from build123d import *

# Parameters (mm, degrees)
BOSS_EXTRUDE2_DEPTH = 6.096


with BuildPart() as part:
    # Sketch1 → Boss-Extrude2 (new body)
    with BuildSketch(Plane.XY):
        with BuildLine():
            Line((-4.0259, 0.692415095), (-4.0259, -1.7018))
            ThreePointArc((-4.0259, -1.7018), (-3.058766591, -4.036666591), (-0.7239, -5.0038))
            Line((-0.7239, -5.0038), (0.7239, -5.0038))
            ThreePointArc((0.7239, -5.0038), (3.058766591, -4.036666591), (4.0259, -1.7018))
            Line((4.0259, -1.7018), (4.0259, 0.692415095))
            ThreePointArc((4.0259, 0.692415095), (3.977581548, 1.682110135), (3.833085773, 2.662391684))
            add(Edge.make_bspline(
                [(3.833085773, 2.662391684), (2.882993145, 7.469428366), (1.294052888, 17.736271143), (0.32760263, 29.308652747), (0, 35.421228256)],
                knots=[0.032373922, 0.032373922, 0.032373922, 0.032373922, 0.516186961, 1, 1, 1, 1], degree=3))
            add(Edge.make_bspline(
                [(-3.833085773, 2.662391684), (-2.882993145, 7.469428366), (-1.294052888, 17.736271143), (-0.32760263, 29.308652747), (0, 35.421228256)],
                knots=[0.032373922, 0.032373922, 0.032373922, 0.032373922, 0.516186961, 1, 1, 1, 1], degree=3))
            ThreePointArc((-3.833085773, 2.662391684), (-3.977581548, 1.682110135), (-4.0259, 0.692415095))
        make_face()
        with BuildLine():
            Line((-1.7399, 1.7018), (-1.7399, -1.7018))
            ThreePointArc((-1.7399, -1.7018), (-1.44232049, -2.42022049), (-0.7239, -2.7178))
            Line((-0.7239, -2.7178), (0.7239, -2.7178))
            ThreePointArc((0.7239, -2.7178), (1.44232049, -2.42022049), (1.7399, -1.7018))
            Line((1.7399, -1.7018), (1.7399, 1.7018))
            ThreePointArc((1.7399, 1.7018), (1.44232049, 2.42022049), (0.7239, 2.7178))
            Line((0.7239, 2.7178), (-0.7239, 2.7178))
            ThreePointArc((-0.7239, 2.7178), (-1.44232049, 2.42022049), (-1.7399, 1.7018))
        make_face(mode=Mode.SUBTRACT)
    extrude(amount=BOSS_EXTRUDE2_DEPTH)


solid = part.part
The model under review builds one solid part; all positions refer to its coordinate system, in mm. A direction names the side the tool comes from. Coordinates: 2 decimals unless noted, no trailing zeros. Answer in a Markdown table with one row per item.
(1) Machinability: for faces 1 (the flat face through (0, 11, 6.096)), 2 (the flat face through (0, 2.718, 3)), which of the approach directions +Z, -Z, +X, -X, +Y, -Y give a long, thin tool a straight path to every point of the face, cutting with its end or side? Answer none if there is none.
Answers:
| item | result |
|---|---|
| face 1 | +Z, +X, -X, +Y, -Y |
| face 2 | +Z, -Z |
(2) Wall thickness on line 1 along X through (y, z) = (1, 5.75); line 2 along X through (y, z) = (16, 3.5); line 3 along X through (y, z) = (20.5, 0.5): over which ranges is each line inside the solid? List them lowest first.
Answers:
| item | result |
|---|---|
| line 1 | -4.02 to -1.74, 1.74 to 4.02 |
| line 2 | -1.7 to 1.7 |
| line 3 | -1.18 to 1.18 |
(3) Insertion check: pin 1 (1 mm diameter, centred on x = -2.5, z = 0.5, fed in from -Y); pin 2 (2 mm diameter, centred on y = 29.5, z = 4, fed in from +X); pin 3 (1 mm diameter, centred on y = 22, z = 5.5, fed in from -X). Each pin has a flat end and moves straight along its axis. Give the tip position at first contact, or say it passes through.
Answers:
| item | result |
|---|---|
| pin 1 | y = -4.75 |
| pin 2 | x = 0.45 |
| pin 3 | x = -1.07 |
(4) The part is to be moulded in two halves that separate along X. For faces 3 (the cylindrical face through (-3.976, 1.696, 3.005)), 4 (the flat face through (-1.74, 0, 3)), 5 (the flat face through (0, -5.004, 3)), say which applies: +X half, -X half, draft (parallel to the pull), parting line (faces both ways), or undercut.
Answers:
| item | result |
|---|---|
| face 3 | -X half |
| face 4 | undercut |
| face 5 | draft |
